Source: CAD feature listing. Evaluate the final solid. Frame: model axes, mm. Give positions to 0.01 mm unless a question says otherwise; leave off trailing zeros. Order: outer loops, then holes, each group sorted by start corner. A loop starts at its lowest first (then second) coordinate and runs counter-clockwise, first axis right, second up. Notation, with made-up numbers: (14, 38.5) -> (35, 38.5) arc R34 cw to (35, 69.5) -> close; hole circle Ø11 at (6, 59.5). An arc over 180 degrees is marked (long way). Answer in a Markdown table with one row per item.
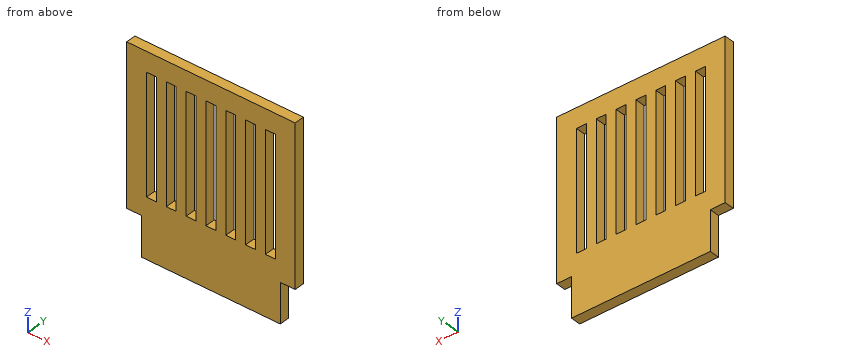
```python
from build123d import *

# Parameters (mm, degrees)
EXTRUDE_1_DEPTH     = 1
SKETCH_5_W          = 1
SKETCH_5_H          = 12
CUT_EXTRUDE_2_DEPTH = 2


with BuildPart() as part:
    # 草图1 → 凸台-拉伸1 (new body)
    with BuildSketch(Plane(origin=(0, 0, 0), x_dir=(1, 0, 0), z_dir=(0, 1, 0))):
        Polygon((-8.5, -8), (-8.5, 8), (-7, 8), (-7, 12), (7, 12), (7, 8), (8.5, 8), (8.5, -8), align=None)
    extrude(amount=EXTRUDE_1_DEPTH)

    # 草图5 → 切除-拉伸2 (cut, through all)
    with BuildSketch(Plane(origin=(0, 1, 0), x_dir=(1, 0, 0), z_dir=(0, 1, 0))):
        Rectangle(SKETCH_5_W, SKETCH_5_H)
        with Locations((2, 0)):
            Rectangle(SKETCH_5_W, SKETCH_5_H)
        with Locations((6, 0)):
            Rectangle(SKETCH_5_W, SKETCH_5_H)
        with Locations((4, 0)):
            Rectangle(SKETCH_5_W, SKETCH_5_H)
        with Locations((-2, 0)):
            Rectangle(SKETCH_5_W, SKETCH_5_H)
        with Locations((-4, 0)):
            Rectangle(SKETCH_5_W, SKETCH_5_H)
        with Locations((-6, 0)):
            Rectangle(SKETCH_5_W, SKETCH_5_H)
    extrude(amount=-CUT_EXTRUDE_2_DEPTH, mode=Mode.SUBTRACT)


solid = part.part
```
(1) Section query A-A (x = -0.25). Return the cut outline in (y, z).
A:
| item | result |
|---|---|
| outline | (0, -12) -> (1, -12) -> (1, -6) -> (0, -6) -> close; (0, 6) -> (1, 6) -> (1, 8) -> (0, 8) -> close |
(2) Ray query, probe 1 along X at (y, z) = (0.95, -10.5). Return the intervals inside material, ascending.
A:
| item | result |
|---|---|
| probe 1 | x = -7 to 7 |
(3) Section query B-B (z = 1.75). Give the number of separate pieces and of enclosed holes in the cut face, plus the area to 3 significant figures.
A:
| item | result |
|---|---|
| separate pieces | 8 |
| enclosed holes | 0 |
| area | 10.0 mm^2 |
